from build123d import *

# Parameters (mm, degrees)
SKETCH1_R           = 6.35
SKETCH1_R_2         = 3.302
BOSS_EXTRUDE1_DEPTH = 5.08
SKETCH2_W           = 12.7
SKETCH2_H           = 12.7
BOSS_EXTRUDE2_DEPTH = 2.54


with BuildPart() as part:
    # Sketch1 → Boss-Extrude1 (new body)
    # profile 1 of 2: a face of its own
    with BuildSketch(Plane.XY):
        Circle(SKETCH1_R)
        Circle(SKETCH1_R_2, mode=Mode.SUBTRACT)
    # profile 2 of 2: a face of its own
    with BuildSketch(Plane.XY):
        with BuildLine():
            ThreePointArc((-3.175, 5.499261314), (0, 6.35), (3.175, 5.499261314))
            Line((3.175, 5.499261314), (3.175, 41.059261314))
            Line((3.175, 41.059261314), (-3.175, 41.059261314))
            Line((-3.175, 41.059261314), (-3.175, 5.499261314))
        make_face()
    extrude(amount=BOSS_EXTRUDE1_DEPTH)

    # Sketch2 → Boss-Extrude2 (add)
    with BuildSketch(Plane(origin=(0, 41.059261314, 0), x_dir=(1, 0, 0), z_dir=(0, 1, 0))):
        with Locations((0, -2.767803864)):
            Rectangle(SKETCH2_W, SKETCH2_H)
    extrude(amount=BOSS_EXTRUDE2_DEPTH)


solid = part.part
Design review of the part built by this model. Coordinates are the model's own, in mm. A direction names the side the tool comes from. Coordinates: 2 decimals unless noted, no trailing zeros. Write each loop counter-clockwise with the first axis right and the second up, starting at its lowest first coordinate (ties: lowest second). Pieces come first, ordered by that corner, then holes. Notation, with made-up numbers: (28, 37) -> (47, 37) arc R35 cw to (47, 69) -> close; hole circle Ø1 at (85, 50.5). An arc over 180 degrees is marked (long way). Write each question's results on one line, items separated by ' | '. Start each with the question number.
(1) For line 1 along Y through (x, z) = (0, 4); line 2 along Z through (x, y) = (-2.5, 23.5); line 3 along X through (y, z) = (40.5, 1.25) (3 decimals), list the stretches that pass through material, from the lowest coordinate up. Write a range as from..to.
(2) Clearance check with flat-ended pins moving along their axes: P1, Ø1.5, axis at y = 20.5, z = 2.5, coming from the +X side (3 decimals); P2, Ø4, axis at x = -1.5, z = 6.5, coming from the -Y side; P3, Ø2, axis at x = -3.5, y = 37.5, coming from the -Z side; P4, Ø6, axis at x = -4.5, y = 2, coming from the +Z side. State where each tip first meets the part, or that it passes through.
(3) Tool access review of faces 5 (the face through (0, 18, 5.08)), 6 (the face through (0, 18, 0)), 7 (the face through (6.35, 42, 3)): name each direction out of +Z, -Z, +X, -X, +Y, -Y from which nothing blocks a thin tool from reaching the whole face with its end or side.
(4) Take a section at B-B on x = 0. Write out the cut boundary in (y, z), and give its area (3 significant figures).
(5) Take a section at C-C on y = 0. Write out the cut boundary in (x, z), and give its area (3 significant figures).
(6) Take a section at D-D on z = -1.25. Write out the cut boundary in (x, y).
(7) The part is to be moulded in two halves that separate along X. For faces 1 (the face through (3.05, -1.26, 2.5)), 2 (the face through (0, 42, 9.118)), 3 (the face through (3.175, 23, 3)), 4 (the face through (-3.175, 24, 3)), say which applies: pulls with the +X half, pulls with the -X half, needs draft (parallel to the pull), parting line crosses it, or undercut.
(8) Take a section at A-A on z = 2.25. Write out the cut boundary in (x, y) (3 decimals), and give its area (3 significant figures).
Results found:
1) line 1: y = -6.35..-3.3, 3.3..43.6 | line 2: z = 0..5.08 | line 3: x = -3.175..3.175
2) P1: stops at x = 3.175 | P2: stops at y = -6.35 | P3: stops at z = 0 | P4: stops at z = 5.08
3) face 5: +Z, +X, -X, -Y | face 6: -Z, +X, -X, -Y | face 7: +Z, -Z, +X, +Y, -Y
4) outline: (-6.35, 0) -> (-3.3, 0) -> (-3.3, 5.08) -> (-6.35, 5.08) -> close; (3.3, 0) -> (41.06, 0) -> (41.06, -3.58) -> (43.6, -3.58) -> (43.6, 9.12) -> (41.06, 9.12) -> (41.06, 5.08) -> (3.3, 5.08) -> close | area: 240 mm2
5) outline: (-6.35, 0) -> (-3.3, 0) -> (-3.3, 5.08) -> (-6.35, 5.08) -> close; (3.3, 0) -> (6.35, 0) -> (6.35, 5.08) -> (3.3, 5.08) -> close | area: 31.0 mm2
6) outline: (-6.35, 41.06) -> (6.35, 41.06) -> (6.35, 43.6) -> (-6.35, 43.6) -> close
7) face 1: undercut | face 2: needs draft | face 3: pulls with the +X half | face 4: pulls with the -X half
8) outline: (-6.35, 41.059) -> (-3.175, 41.059) -> (-3.175, 5.499) arc R6.35 ccw (long way) to (3.175, 5.499) -> (3.175, 41.059) -> (6.35, 41.059) -> (6.35, 43.599) -> (-6.35, 43.599) -> close; hole circle Ø6.604 at (0, 0) | area: 347 mm2
